CAD build for the part. Positions are in the model's coordinates, mm. A direction names the side the tool comes from. Coordinates: 2 decimals unless noted, no trailing zeros. Order: outer loops, then holes, each group sorted by start corner. A loop starts at its lowest first (then second) coordinate and runs counter-clockwise, first axis right, second up.
from build123d import *

# Parameters (mm, degrees)
F1_DEPTH       = 20
F3_DEPTH       = 40
F5_D           = 6.5
F5_START       = 0.4050409
F5_CSINK_D     = 9
F5_CSINK_ANGLE = 90
F8_D           = 6.5
F8_START       = 1.0000001
F8_CSINK_D     = 12.5
F8_CSINK_ANGLE = 90


with BuildPart() as f1:
    # F0 (on Top) → F1 (new body)
    with BuildSketch(Plane.XY):
        with BuildLine():
            ThreePointArc((-20, 12), (-32, 0), (-20, -12))
            Line((-20, -12), (20, -12))
            ThreePointArc((20, -12), (32, 0), (20, 12))
            Line((20, 12), (-20, 12))
        make_face()
    extrude(amount=F1_DEPTH)

    # F2 (on Right) → F3 (intersect, symmetric)
    with BuildSketch(Plane.YZ):
        with BuildLine():
            ThreePointArc((15, 10.218678296), (0, 4), (-15, 10.218678296))
            Line((-15, 10.218678296), (-15, 4.9505555632))
            ThreePointArc((-15, 4.9505555632), (0, 0), (15, 4.9505555632))
            Line((15, 4.9505555632), (15, 10.218678296))
        make_face()
    extrude(amount=F3_DEPTH, both=True, mode=Mode.INTERSECT)

    # F5 (through all)
    # its depths count from where the whole tool has entered the part; down to there all is cleared
    with Locations(Plane(origin=(0, 0, 0), x_dir=(1, 0, 0), z_dir=(0, 0, -1)).offset(-F5_START)):
        with Locations((-21.5, 0), (21.5, 0)):
            CounterSinkHole(F5_D / 2, F5_CSINK_D / 2, counter_sink_angle=F5_CSINK_ANGLE)

    # F8 (through all)
    # its depths count from where the whole tool has entered the part; down to there all is cleared
    with Locations(Plane.XY.offset(5).offset(-F8_START)):
        with Locations((0, 0)):
            CounterSinkHole(F8_D / 2, F8_CSINK_D / 2, counter_sink_angle=F8_CSINK_ANGLE)


solid = f1.part
1) Slice it at B-B (y = -0.75). Give the number of separate pieces and of enclosed holes in the cut face, plus the area to 3 significant figures.
2) Which spindle directions (+Z, -Z, +X, -X, +Y, -Y) get a long thin tool onto all of the face, cutting with end or side? Do faces 1 (the cylindrical face through (-17, 0.1, 0.2)), 2 (the cylindrical face through (0.14, 6.25, 4.37)), 3 (the cylindrical face through (0.448, 5.343, 0.573)). Say none if no direction does.
3) Pin check, flat tips, straight feed: P1, Ø3, axis at x = -4.5, y = -6, coming from the +Z side; P2, Ø6, axis at x = -2, y = 3.5, coming from the +Z side; P3, Ø3, axis at x = -22.5, z = 6.5, coming from the +Y side; P4, Ø4, axis at x = 21.5, y = 0, coming from the -Z side. Stop position of each tip, or through.
4) Slice it at C-C (x = 14). List the corners of the cut face in (y, z).
5) Slice it at A-A (x = 0). List the corners of the cut face in (y, z).
6) Drill centre lines: probe 1 along X at (y, z) = (0, 0.3); probe 2 along X at (y, z) = (1.25, 2); probe 3 along Z at (x, y) = (-26.5, 0.5). Where is each one in solid material? Low to high.
7) Slice it at D-D (y = -10). List the corners of the cut face in (x, z), plus the area to 3 significant figures.
Worked out:
1. separate pieces: 4
1. enclosed holes: 0
1. area: 166 mm2
2. face 1: -Z
2. face 2: +Z
2. face 3: -Z, +X, -X
3. P1: stops at z = 5.37
3. P2: stops at z = 5.02
3. P3: stops at y = 11.96
3. P4: passes through
4. outline: (-12, 3.04) arc R25.2 ccw to (12, 3.04) - (12, 7.72) arc R21.2 cw to (-12, 7.72) - close
5. outline: (-12, 3.04) arc R25.2 ccw to (-3.25, 0.21) - (-3.25, 1) - (-6.25, 4) - (-6.25, 4.94) arc R21.2 cw to (-12, 7.72) - close; (3.25, 0.21) arc R25.2 ccw to (12, 3.04) - (12, 7.72) arc R21.2 cw to (6.25, 4.94) - (6.25, 4) - (3.25, 1) - close
6. probe 1: x = -32 to -26, -17 to -3.25, 3.25 to 17, 26 to 32
6. probe 2: x = -31.93 to -24.5, -18.5 to -4.06, 4.06 to 18.5, 24.5 to 31.93
6. probe 3: z = 0 to 4.01
7. outline: (-26.63, 2.07) - (26.63, 2.07) - (26.63, 6.51) - (-26.63, 6.51) - close
7. area: 236 mm2
